Can you work these out from the model? Positions are in its coordinate system, mm. A direction names the side the tool comes from. Give positions to 0.01 mm unless a question says otherwise; leave off trailing zeros. Loops run counter-clockwise (first coordinate to the right, second up) from the corner with the lowest first, then second, coordinate; pieces in that order, holes last. Notation, with made-up numbers: (60.5, 61.25) - (94.5, 61.25) arc R18 cw to (94.5, 72.25) - close; hole circle Ø10 at (-37.75, 1). An arc over 180 degrees is marked (long way). Answer as a JSON object with one key per item and string values.
```python
from build123d import *

# Parameters (mm, degrees)
SKETCH1_R               = 28
BOSS_EXTRUDE1_DEPTH     = 5
SKETCH2_R               = 23
BOSS_EXTRUDE2_DEPTH     = 4.7625
SKETCH3_R               = 20
CUT_EXTRUDE1_DEPTH      = 1
CUT_EXTRUDE1_DEPTH_BACK = 10.7625


with BuildPart() as part:
    # Sketch1 → Boss-Extrude1 (new body)
    with BuildSketch(Plane.XY):
        Circle(SKETCH1_R)
    extrude(amount=BOSS_EXTRUDE1_DEPTH)

    # Sketch2 → Boss-Extrude2 (add)
    with BuildSketch(Plane.XY.offset(5)):
        Circle(SKETCH2_R)
    extrude(amount=BOSS_EXTRUDE2_DEPTH)

    # Sketch3 → Cut-Extrude1 (cut, two sides)
    with BuildSketch(Plane.XY.offset(9.7625)) as cut_extrude1_sk:
        Circle(SKETCH3_R)
    extrude(amount=CUT_EXTRUDE1_DEPTH, mode=Mode.SUBTRACT)
    extrude(cut_extrude1_sk.sketch, amount=-CUT_EXTRUDE1_DEPTH_BACK, mode=Mode.SUBTRACT)


solid = part.part
```
1) I'm going to push flat-ended pins straight in: P1, Ø2, axis at y = -13.5, z = 8.5, coming from the -X side; P2, Ø4, axis at y = 11.5, z = 4, coming from the -X side; P3, Ø2, axis at x = -17, z = 7.5, coming from the -Y side. Where does each tip first touch, or does it pass through?
Check sheet entries:
{"P1": "x = -19.31", "P2": "x = -26.34", "P3": "y = -16.52"}
2) Imagine slicing it at A-A on x = 0. Write out the boundary of the cut face in (y, z), and give its area (3 significant figures).
Check sheet entries:
{"outline": "(-28, 0) - (-20, 0) - (-20, 9.76) - (-23, 9.76) - (-23, 5) - (-28, 5) - close; (20, 0) - (28, 0) - (28, 5) - (23, 5) - (23, 9.76) - (20, 9.76) - close", "area": "109 mm2"}
3) I need wall thicknesses on L1, parallel to Y at x = 0, z = 3; L2, parallel to Y at x = 0, z = 7.25; L3, parallel to X at y = -10, z = 7. Which ranges of each line are inside material? Lowest first, please.
Check sheet entries:
{"L1": "-28 to -20, 20 to 28", "L2": "-23 to -20, 20 to 23", "L3": "-20.71 to -17.32, 17.32 to 20.71"}
4) Imagine slicing it at C-C on z = 3.25. Write out the boundary of the cut face in (x, y), and give its area (3 significant figures).
Check sheet entries:
{"outline": "circle Ø56 at (0, 0); hole circle Ø40 at (0, 0)", "area": "1,210 mm2"}
5) Imagine slicing it at D-D on z = 9. Write out the boundary of the cut face in (x, y).
Check sheet entries:
{"outline": "circle Ø46 at (0, 0); hole circle Ø40 at (0, 0)"}
6) If we mould it in two halves opening along X, with no side actions, what happens to faces 3 (the cylindrical face through (-4.336, -19.524, 4.95)), 4 (the cylindrical face through (25.865, -10.724, 2.465)), 5 (the flat face through (-7, 19, 9.762))? For each: released by +X, released by -X, zero draft, split by the parting line, or undercut.
Check sheet entries:
{"face 3": "undercut", "face 4": "split by the parting line", "face 5": "zero draft"}
7) Which directions (+Z, -Z, +X, -X, +Y, -Y) give clear straight access to the entire face, cutting with the end or side of a thin tool? Please do faces 1 (the flat face through (-7, 19, 0)), 2 (the cylindrical face through (-2.994, 22.804, 7.348)).
Check sheet entries:
{"face 1": "-Z, +X, -X, +Y, -Y", "face 2": "+Z"}
